```python
from build123d import *

# Parameters (mm, degrees)
F0_R     = 17.78
F0_W     = 48.26
F0_H     = 38.1
F0_R_2   = 7.62
F1_DEPTH = 12.7
F5_W     = 48.26
F5_H     = 38.1
F6_DEPTH = 10.922
F7_R     = 3.81
F8_R     = 1.27
F9_R     = 0.762


with BuildPart() as f1:
    # F0 (on Front) → F1 (new body)
    with BuildSketch(Plane.XZ):
        with BuildLine():
            Line((24.13, 44.45), (-24.13, 44.45))
            ThreePointArc((-24.13, 44.45), (-28.620128, 42.590128), (-30.48, 38.1))
            Line((-30.48, 38.1), (-30.48, -53.34))
            ThreePointArc((-30.48, -53.34), (-28.620128, -57.830128), (-24.13, -59.69))
            Line((-24.13, -59.69), (24.13, -59.69))
            ThreePointArc((24.13, -59.69), (28.620128, -57.830128), (30.48, -53.34))
            Line((30.48, -53.34), (30.48, 38.1))
            ThreePointArc((30.48, 38.1), (28.620128, 42.590128), (24.13, 44.45))
        make_face()
        with Locations((0, -29.21)):
            Circle(F0_R, mode=Mode.SUBTRACT)
        with Locations((0, 19.05)):
            Rectangle(F0_W, F0_H, mode=Mode.SUBTRACT)
        with Locations((0, -29.21)):
            Circle(F0_R)
        with Locations((0, -29.21)):
            Circle(F0_R_2, mode=Mode.SUBTRACT)
        with Locations((0, -29.21)):
            Circle(F0_R_2)
    extrude(amount=F1_DEPTH)

    # F3 (on Right) → F4 (revolve, cut)
    with BuildSketch(Plane.YZ):
        Polygon((-16.624968, -29.21), (-10.382934, -29.21), (-10.382934, -21.59), (-12.636651, -11.43), (-16.624968, -11.43), align=None)
    revolve(axis=Axis((0, -8.021076, -29.21), (0, 1, 0)), mode=Mode.SUBTRACT)

    # F5 (on Front) → F6 (join)
    with BuildSketch(Plane.XZ):
        with Locations((0, 19.05)):
            Rectangle(F5_W, F5_H)
    extrude(amount=F6_DEPTH)

    # F7
    f7_edges = [f1.edges().sort_by_distance(p)[0] for p in [
        (28.620128, 0, 42.590128),
    ]]
    fillet(f7_edges, radius=F7_R)

    # F8
    f8_edges = [f1.edges().sort_by_distance(p)[0] for p in [
        (28.620128, -12.7, 42.590128),
    ]]
    fillet(f8_edges, radius=F8_R)

    # F9
    f9_edges = [f1.edges().sort_by_distance(p)[0] for p in [
        (0, -12.7, 0),
        (-24.13, -12.7, 19.05),
        (0, -12.7, 38.1),
        (24.13, -12.7, 19.05),
    ]]
    fillet(f9_edges, radius=F9_R)


solid = f1.part
```
For this review, take the finished solid that the model builds, in its own axes (mm). A direction names the side the tool comes from. Give positions to 0.01 mm unless a question says otherwise; leave off trailing zeros. Write each loop counter-clockwise with the first axis right and the second up, starting at its lowest first coordinate (ties: lowest second). Pieces come first, ordered by that corner, then holes.
Item 1: Take a section at A-A (z = 11). Give the boundary of the cut face in (x, y).
Item 2: Wall thickness on probe 1 along Y at (x, z) = (-24, -0.5); probe 2 along Y at (x, z) = (19, 2.5); probe 3 along X at (y, z) = (-12, 11): over which ranges is each line inside the solid? List them lowest first.
Item 3: Take a section at B-B (x = 0). Give the boundary of the cut face in (y, z), and give its area (3 significant figures).
Item 4: Machinability: for faces 1 (the face through (0, -10.922, 19)), 2 (the face through (0, -12.7, -7)), which of the approach directions +Z, -Z, +X, -X, +Y, -Y give a long, thin tool a straight path to every point of the face, cutting with its end or side? Answer none if there is none.
Item 5: Take a section at C-C (z = -29.21). Give the boundary of the cut face in (x, y), and give its area (3 significant figures).
Item 6: The part is to be moulded in two halves that separate along Z. For faces 3 (the face through (28.67, -7.57, 42.54)), 4 (the face through (0, -10.383, -29)), 5 (the face through (0, 0, -7)), say which applies: +Z half, -Z half, draft (parallel to the pull), parting line (faces both ways), or undercut.
Item 7: Insertion check: P1, Ø11.5, axis at x = -6.5, z = 27, coming from the -Y side; P2, Ø1.5, axis at x = 2, z = -21, coming from the -Y side; P3, Ø1.5, axis at y = -2, z = -38, coming from the +X side. Each pin has a flat end and moves straight along its axis. Give the tip position at first contact, or say it passes through.
Established:
1. outline: (-30.48, -11.43) arc R1.27 ccw to (-29.21, -12.7) - (-24.89, -12.7) arc R0.76 ccw to (-24.13, -11.94) - (-24.13, -10.92) - (24.13, -10.92) - (24.13, -11.94) arc R0.76 ccw to (24.89, -12.7) - (29.21, -12.7) arc R1.27 ccw to (30.48, -11.43) - (30.48, -3.81) arc R3.81 ccw to (26.67, 0) - (-26.67, 0) arc R3.81 ccw to (-30.48, -3.81) - close
2. probe 1: y = -12.65 to 0
2. probe 2: y = -10.92 to 0
2. probe 3: x = -30.34 to -24.13, 24.13 to 30.34
3. outline: (-12.7, -58.42) arc R1.27 ccw to (-11.43, -59.69) - (-3.81, -59.69) arc R3.81 ccw to (0, -55.88) - (0, 40.64) arc R3.81 ccw to (-3.81, 44.45) - (-11.43, 44.45) arc R1.27 ccw to (-12.7, 43.18) - (-12.7, 38.86) arc R0.76 ccw to (-11.94, 38.1) - (-10.92, 38.1) - (-10.92, 0) - (-11.94, 0) arc R0.76 ccw to (-12.7, -0.76) - (-12.7, -11.43) - (-12.64, -11.43) - (-10.38, -21.59) - (-10.38, -36.83) - (-12.64, -46.99) - (-12.7, -46.99) - close
3. area: 1,190 mm2
4. face 1: -Y
4. face 2: +Z, -Z, +X, -X, -Y
5. outline: (-30.48, -11.43) arc R1.27 ccw to (-29.21, -12.7) - (-17.78, -12.7) - (-17.78, -12.64) - (-7.62, -10.38) - (7.62, -10.38) - (17.78, -12.64) - (17.78, -12.7) - (29.21, -12.7) arc R1.27 ccw to (30.48, -11.43) - (30.48, -3.81) arc R3.81 ccw to (26.67, 0) - (-26.67, 0) arc R3.81 ccw to (-30.48, -3.81) - close
5. area: 708 mm2
6. face 3: +Z half
6. face 4: undercut
6. face 5: draft
7. P1: stops at y = -10.92
7. P2: stops at y = -10.73
7. P3: stops at x = 30.33
